from build123d import *

# Parameters (mm, degrees)
BOSS_EXTRUDE2_DEPTH  = 21
FILLET1_R            = 5
SKETCH4_R            = 0.5
BOSS_EXTRUDE3_DEPTH  = 21
SKETCH5_R            = 0.5
BOSS_EXTRUDE4_DEPTH  = 21
FILLET2_R            = 1
BOSS_EXTRUDE5_DEPTH  = 1.5
FILLET3_R            = 1
FILLET4_R            = 1
SKETCH7_R            = 0.5
BOSS_EXTRUDE6_DEPTH  = 3
SKETCH8_W            = 3
SKETCH8_H            = 7
BOSS_EXTRUDE7_DEPTH  = 1.5
FILLET5_R            = 1
SKETCH9_R            = 0.5
BOSS_EXTRUDE8_DEPTH  = 3
SKETCH10_W           = 10
SKETCH10_H           = 17
CUT_EXTRUDE1_DEPTH   = 36.951356024
CUT_EXTRUDE2_DEPTH   = 41.880924647
SKETCH12_W           = 18
SKETCH12_H           = 21
SKETCH12_W_2         = 10
SKETCH12_H_2         = 17
BOSS_EXTRUDE9_DEPTH  = 10
BOSS_EXTRUDE10_DEPTH = 10
BOSS_EXTRUDE14_DEPTH = 10
BOSS_EXTRUDE15_DEPTH = 10
LPATTERN1_START      = 2
LPATTERN1_DEPTH      = 10
SKETCH17_W           = 2.875504222
SKETCH17_H           = 35
BOSS_EXTRUDE16_DEPTH = 10
BOSS_EXTRUDE17_DEPTH = 10
FILLET6_R            = 1
FILLET7_R            = 1
FILLET8_R            = 1
FILLET9_R            = 2


# Read off the part's stored shape, not the designer's step: LPattern1
with BuildPart() as part:
    # Sketch3 → Boss-Extrude2 (new body)
    with BuildSketch(Plane(origin=(0, 0, 0), x_dir=(1, 0, 0), z_dir=(0, 1, 0))):
        Polygon((0, 0), (-5.5, 5.5), (-5.5, 18), (-7.5, 18), (-7.5, 3.5), (-2, -2), (16, -2), (21.5, 3.5), (21.5, 18), (19.5, 18), (19.5, 5.5), (14, 0), align=None)
    extrude(amount=BOSS_EXTRUDE2_DEPTH)

    # Fillet1
    fillet1_edges = [part.edges().sort_by_distance(p)[0] for p in [
        (-7.5, 10.5, -3.5),
        (21.5, 10.5, -3.5),
    ]]
    fillet(fillet1_edges, radius=FILLET1_R)

    # Sketch4 → Boss-Extrude3 (add)
    with BuildSketch(Plane(origin=(0, 21, 0), x_dir=(1, 0, 0), z_dir=(0, 1, 0))):
        with Locations((-5.5, 17.5)):
            Circle(SKETCH4_R)
    extrude(amount=-BOSS_EXTRUDE3_DEPTH)

    # Sketch5 → Boss-Extrude4 (add)
    with BuildSketch(Plane(origin=(0, 21, 0), x_dir=(1, 0, 0), z_dir=(0, 1, 0))):
        with Locations((19.5, 17.5)):
            Circle(SKETCH5_R)
    extrude(amount=-BOSS_EXTRUDE4_DEPTH)

    # Fillet2
    fillet2_edges = [part.edges().sort_by_distance(p)[0] for p in [
        (-7.5, 10.5, -18),
        (21.5, 10.5, -18),
    ]]
    fillet(fillet2_edges, radius=FILLET2_R)

    # Sketch6 → Boss-Extrude5 (add)
    with BuildSketch(Plane(origin=(0, 21, 0), x_dir=(1, 0, 0), z_dir=(0, 1, 0))):
        Polygon((1.451426333, 5), (1.451426333, 0), (1.451426333, -2), (4.451426333, -2), (4.451426333, 0), (4.451426333, 5), align=None)
    extrude(amount=BOSS_EXTRUDE5_DEPTH)

    # Fillet3
    fillet3_edges = [part.edges().sort_by_distance(p)[0] for p in [
        (2.951426333, 22.5, 2),
    ]]
    fillet(fillet3_edges, radius=FILLET3_R)

    # Fillet4
    fillet4_edges = [part.edges().sort_by_distance(p)[0] for p in [
        (2.951426333, 22.5, -5),
    ]]
    fillet(fillet4_edges, radius=FILLET4_R)

    # Sketch7 → Boss-Extrude6 (add)
    with BuildSketch(Plane.ZY.offset(-1.451426333)):
        with Locations((-4.5, 21)):
            Circle(SKETCH7_R)
    extrude(amount=-BOSS_EXTRUDE6_DEPTH)

    # Sketch8 → Boss-Extrude7 (add)
    with BuildSketch(Plane.XZ):
        with Locations((2.951426333, -1.5)):
            Rectangle(SKETCH8_W, SKETCH8_H)
    extrude(amount=BOSS_EXTRUDE7_DEPTH)

    # Fillet5
    fillet5_edges = [part.edges().sort_by_distance(p)[0] for p in [
        (2.951426333, -1.5, -5),
        (2.951426333, -1.5, 2),
    ]]
    fillet(fillet5_edges, radius=FILLET5_R)

    # Sketch9 → Boss-Extrude8 (add)
    with BuildSketch(Plane(origin=(4.451426333, 0, 0), x_dir=(0, 0, -1), z_dir=(1, 0, 0))):
        with Locations((4.5, 0)):
            Circle(SKETCH9_R)
    extrude(amount=-BOSS_EXTRUDE8_DEPTH)

    # Sketch10 → Cut-Extrude1 (cut, through all)
    with BuildSketch(Plane(origin=(0, 0, 0), x_dir=(-1, 0, 0), z_dir=(0, 0, -1))):
        with Locations((-7, 10.5)):
            Rectangle(SKETCH10_W, SKETCH10_H)
    extrude(amount=-CUT_EXTRUDE1_DEPTH, mode=Mode.SUBTRACT)

    # Sketch11 → Cut-Extrude2 (cut, through all)
    with BuildSketch(Plane.ZY.offset(7.5)):
        Polygon((-6.571067812, 19.4), (-6.571067812, 1.604815424), (-15.4686601, 10.502407712), align=None)
    extrude(amount=-CUT_EXTRUDE2_DEPTH, mode=Mode.SUBTRACT)

    # Sketch12 → Boss-Extrude9 (add)
    with BuildSketch(Plane.XY.offset(2)):
        with Locations((7, 10.5)):
            Rectangle(SKETCH12_W, SKETCH12_H)
        with Locations((7, 10.5)):
            Rectangle(SKETCH12_W_2, SKETCH12_H_2, mode=Mode.SUBTRACT)
    extrude(amount=BOSS_EXTRUDE9_DEPTH)

    # Sketch13 → Boss-Extrude10 (add)
    with BuildSketch(Plane.XY.offset(12)):
        Polygon((16, 21), (-34, 99), (-34, 70.921750355), (-2, 21), align=None)
        Polygon((-0.906392677, 23), (-32, 71.507728201), (-32, 92.174004857), (12.342310806, 23), align=None, mode=Mode.SUBTRACT)
    extrude(amount=-BOSS_EXTRUDE10_DEPTH)

    # Sketch14 → Boss-Extrude14 (add)
    with BuildSketch(Plane.XY.offset(12)):
        Polygon((10.585384641, 25.740804817), (-4.823944827, 29.111595638), (-6.748576082, 29.532608725), (-6.534879203, 30.509508743), (-4.610247948, 30.088495656), (10.79908152, 26.717704835), align=None)
    extrude(amount=-BOSS_EXTRUDE14_DEPTH)

    # Sketch16 → Boss-Extrude15 (add)
    with BuildSketch(Plane.XY.offset(12)):
        Polygon((-5.587116842, 30.302185726), (-2.216332829, 45.71148407), (-2.025604345, 46.583385709), (-1.775197733, 47.728101652), (-2.75209775, 47.941798531), (-3.002504363, 46.797082588), (-3.193232846, 45.925180949), (-6.564016859, 30.515882605), align=None)
    extrude(amount=-BOSS_EXTRUDE15_DEPTH)

    # LPattern1 outline → LPattern1 (add)
    with BuildSketch(Plane.XY.offset(LPATTERN1_START)):
        Polygon((-2.979535968, 46.902080966), (-3.669471366, 47.978380187), (-19.078219518, 51.349043846), (-18.315047503, 50.158453758), (-3.000050935, 46.808298259), align=None)
        Polygon((-19.078649352, 51.349714409), (-15.707985697, 66.758462544), (-17.161124234, 69.025358662), (-32, 72.271362735), (-32, 71.507728201), (-31.80615018, 71.205311878), (-16.491703803, 67.855276733), (-19.841845682, 52.54034243), align=None)
        Polygon((-32, 75.003788744), (-29.199638565, 87.805441018), (-29.962841704, 88.996037915), (-32, 79.683314274), align=None)
    extrude(amount=LPATTERN1_DEPTH)



with BuildPart() as body_2:
    # Sketch17 → Boss-Extrude16 (new body)
    with BuildSketch(Plane.XY.offset(12)):
        with Locations((-43.437752111, 81.5)):
            Rectangle(SKETCH17_W, SKETCH17_H)
    extrude(amount=-BOSS_EXTRUDE16_DEPTH)


with BuildPart() as part_1:
    add(part.part)

    add(body_2.part)  # Boss-Extrude17 merges body 2
    # Sketch18 → Boss-Extrude17 (add)
    with BuildSketch(Plane.XY.offset(12)):
        Polygon((-34, 64), (-34, 71.035157721), (-31.80615018, 71.205311878), (-31.80615018, 61.08148926), (-34, 61.08148926), (-44.875504222, 61.08148926), (-44.875504222, 64), (-42, 64), align=None)
    extrude(amount=-BOSS_EXTRUDE17_DEPTH)

    # Fillet6
    fillet6_edges = [part_1.edges().sort_by_distance(p)[0] for p in [
        (-31.80615018, 67.499224635, 7),
    ]]
    fillet(fillet6_edges, radius=FILLET6_R)

    # Fillet7
    fillet7_edges = [part_1.edges().sort_by_distance(p)[0] for p in [
        (-34, 99, 7),
        (-44.875504222, 61.08148926, 7),
        (-31.80615018, 61.08148926, 7),
        (-42, 99, 7),
        (-44.875504222, 99, 7),
    ]]
    fillet(fillet7_edges, radius=FILLET7_R)

    # Fillet8
    fillet8_edges = [part_1.edges().sort_by_distance(p)[0] for p in [
        (-34, 64, 7),
        (-42, 64, 7),
    ]]
    fillet(fillet8_edges, radius=FILLET8_R)

    # Fillet9
    fillet9_edges = [part_1.edges().sort_by_distance(p)[0] for p in [
        (2, 19, 6),
        (2, 2, 6),
        (12, 2, 6),
        (12, 19, 6),
        (16, 0, 7),
        (16, 21, 7),
        (-2, 21, 7),
        (-2, 0, 7),
    ]]
    fillet(fillet9_edges, radius=FILLET9_R)


solid = part_1.part
The model under review builds one solid part; all positions refer to its coordinate system, in mm. A direction names the side the tool comes from. Round coordinates to 2 decimals unless told otherwise and drop trailing zeros. Write each loop counter-clockwise with the first axis right and the second up, starting at its lowest first coordinate (ties: lowest second). Pieces come first, ordered by that corner, then holes. Notation, with made-up numbers: (-19, -31.5) - (-1, -31.5) arc R19 cw to (-1, -23.5) - close; hole circle Ø8 at (61, 23). An arc over 180 degrees is marked (long way). One line per item, written item: value. Start each with the question number.
1. Consider section D-D on z = 5. State how many separate pieces and enclosed holes the cut face has, and give its area (3 significant figures).
2. Consider section A-A on y = 32.5. Write out the cut boundary in (x, z).
3. Machinability: for faces 1 (the face through (-7, 11, -6.571)), 2 (the face through (17.4, 21, -2.8)), 3 (the face through (6, 23, 7)), 4 (the face through (-1.4, 0.57, 7.07)), which of the approach directions +Z, -Z, +X, -X, +Y, -Y give a long, thin tool a straight path to every point of the face, cutting with its end or side? Answer none if there is none.
4. Consider section C-C on x = -22. Write out the cut boundary in (y, z), and give its area (3 significant figures).
5. Clearance check with flat-ended pins moving along their axes: P1, Ø3, axis at x = 6, z = 7.5, coming from the +Y side; P2, Ø2, axis at y = 21, z = -1, coming from the -X side; P3, Ø4, axis at x = -18, z = 3, coming from the +Y side; P4, Ø8, axis at x = 14.5, y = 33, coming from the -Z side. State where each tip first meets the part, or that it passes through.
6. The part is to be moulded in two halves that separate along Z. For faces 5 (the face through (3.72, 36.45, 7.07)), 6 (the face through (20, 11, -6.571)), say which applies: released by +Z, released by -Z, zero draft, split by the parting line, or undercut.
7. Consider section B-B on y = 84.5. Write out the cut boundary in (x, z), and give its area (3 significant figures).
8. To check wall thickness, follow L1, parallel to X at y = 55.5, z = 8.5; L2, parallel to X at y = 9.5, z = -15.5; L3, parallel to Y at x = -7, z = -6.5. State the ranges of each line that lie inside material, in increasing order. Write a range as from..to.
Checks:
1. separate pieces: 1
1. enclosed holes: 8
1. area: 821 mm^2
2. outline: (-9.37, 2) - (-7, 2) - (-7, 12) - (-9.37, 12) - close; (-6.13, 2) - (-5.11, 2) - (-5.11, 12) - (-6.13, 12) - close; (6.25, 2) - (8.63, 2) - (8.63, 12) - (6.25, 12) - close
3. face 1: +X, -X
3. face 2: -Z, +X, +Y
3. face 3: +Z, -Z
3. face 4: +Z, -X, -Y
4. outline: (52.2, 2) - (55.91, 2) - (55.91, 12) - (52.2, 12) - close; (69.06, 2) - (70.08, 2) - (70.08, 12) - (69.06, 12) - close; (76.57, 2) - (80.28, 2) - (80.28, 12) - (76.57, 12) - close
4. area: 84.4 mm^2
5. P1: stops at y = 38.94
5. P2: stops at x = -6
5. P3: stops at y = 77.16
5. P4: passes through
6. face 5: zero draft
6. face 6: undercut
7. outline: (-44.88, 2) - (-42, 2) - (-42, 12) - (-44.88, 12) - close; (-34, 2) - (-32, 2) - (-32, 12) - (-34, 12) - close; (-30.95, 2) - (-29.92, 2) - (-29.92, 12) - (-30.95, 12) - close; (-27.08, 2) - (-24.71, 2) - (-24.71, 12) - (-27.08, 12) - close
7. area: 82.7 mm^2
8. L1: x = -24.11..-21.74, -19.19..-18.17, -8.49..-6.12
8. L2: x = -7.5..-5.5, 19.5..21.5
8. L3: y = 0..21
